from build123d import *

# Parameters (mm, degrees)
F0_W     = 238.260204
F0_H     = 225.335434
F0_R     = 12.796383
F0_R_2   = 8.036505
F0_R_3   = 6.535103
F0_R_4   = 9.083022
F1_DEPTH = 25


with BuildPart() as f1:
    # F0 (on Front) → F1 (new body)
    with BuildSketch(Plane.XZ):
        with Locations((32.97555, 59.378974)):
            Rectangle(F0_W, F0_H)
        Circle(F0_R, mode=Mode.SUBTRACT)
        with Locations((61.056477, 10.000178)):
            Circle(F0_R_2, mode=Mode.SUBTRACT)
        with Locations((0, 108)):
            Circle(F0_R_3, mode=Mode.SUBTRACT)
        with Locations((61.056535, 98.000178)):
            Circle(F0_R_4, mode=Mode.SUBTRACT)
    extrude(amount=F1_DEPTH)


solid = f1.part
Check sheet for the modelled part. Datum: model origin and axes. Units: mm. Coordinates: 2 decimals unless noted, no trailing zeros. Loops run counter-clockwise (first coordinate to the right, second up) from the corner with the lowest first, then second, coordinate; pieces in that order, holes last. Notation, with made-up numbers: (84.5, 25.5) -> (127.5, 25.5) arc R25 ccw to (127.5, 48.5) -> close; hole circle Ø1 at (75.25, 47.5). An arc over 180 degrees is marked (long way). Write item = value, one per line. Start each with the question number.
1. Section check B-B on y = -8.5. Record the cut outline in (x, z), then the cut area to 3 significant figures.
2. Section check A-A on x = 0. Record the cut outline in (y, z).
3. Draft check along Z on faces 1 (the cylindrical face through (-0.85, -12.32, 114.48)), 2 (the flat face through (31, -25, 61)), 3 (the flat face through (31, -12, 172.047)). Enter one of: released by +Z, released by -Z, zero draft, split by the parting line, or undercut.
4. Depth check by flat-ended pin: P1, Ø23, axis at x = 0, z = 0, coming from the -Y side; P2, Ø2, axis at x = 4.5, z = 90.5, coming from the +Y side. Enter the tip coordinate at first touch or a pass-through.
5. Material ranges on line 1 (Z direction, x = 0, y = -17.75); line 2 (X direction, y = -9, z = 98.5); line 3 (X direction, y = -4.5, z = 10), recorded low to high.
Responses:
q1.outline = (-86.15, -53.29) -> (152.11, -53.29) -> (152.11, 172.05) -> (-86.15, 172.05) -> close; hole circle Ø25.59 at (0, 0); hole circle Ø13.07 at (0, 108); hole circle Ø18.17 at (61.06, 98); hole circle Ø16.07 at (61.06, 10)
q1.area = 52,600 mm2
q2.outline = (-25, -53.29) -> (0, -53.29) -> (0, -12.8) -> (-25, -12.8) -> close; (-25, 12.8) -> (0, 12.8) -> (0, 101.46) -> (-25, 101.46) -> close; (-25, 114.54) -> (0, 114.54) -> (0, 172.05) -> (-25, 172.05) -> close
q3.face_1 = undercut
q3.face_2 = zero draft
q3.face_3 = released by +Z
q4.P1 = through
q4.P2 = 0
q5.line_1 = -53.29 to -12.8, 12.8 to 101.46, 114.54 to 172.05
q5.line_2 = -86.15 to 51.99, 70.13 to 152.11
q5.line_3 = -86.15 to -7.98, 7.98 to 53.02, 69.09 to 152.11
